```python
from build123d import *


with BuildPart() as part:
    # Sketch1 → Revolve1 (revolve)
    with BuildSketch(Plane.XY, mode=Mode.PRIVATE) as revolve1_sk:
        with BuildLine():
            Line((0, 0), (55.850610629, 0))
            ThreePointArc((55.850610629, 0), (64.83086675, 3.719743879), (68.550610629, 12.7))
            Line((68.550610629, 12.7), (68.550610629, 135.537090781))
            ThreePointArc((68.550610629, 135.537090781), (67.07437947, 141.479902659), (62.988876295, 146.041145392))
            Line((62.988876295, 146.041145392), (36.426242146, 164.092378593))
            ThreePointArc((36.426242146, 164.092378593), (33.255344861, 167.632513451), (32.109591896, 172.244930881))
            Line((32.109591896, 172.244930881), (32.109591896, 182.693006016))
            Line((32.109591896, 182.693006016), (37.812538782, 182.693006016))
            Line((37.812538782, 182.693006016), (37.812538782, 191.889991998))
            Line((37.812538782, 191.889991998), (0, 191.889991998))
            Line((0, 191.889991998), (0, 0))
        make_face()
    revolve(revolve1_sk.sketch.rotate(Axis((0, 191.889991998, 0), (0, -1, 0)), 90), axis=Axis((0, 191.889991998, 0), (0, -1, 0)))


solid = part.part
```
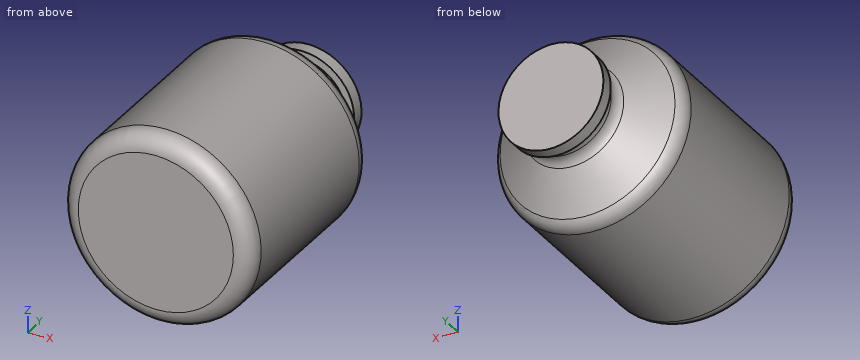
Build history of the part. All positions in model axes, mm. Coordinates: 2 decimals unless noted, no trailing zeros. Order: outer loops, then holes, each group sorted by start corner. A loop starts at its lowest first (then second) coordinate and runs counter-clockwise, first axis right, second up.
Item 1: Saw through at B-B on z = 0. List the corners of the cut face in (x, y), then the cut area to 3 significant figures.
Filled in:
outline: (-68.55, 12.7) arc R12.7 ccw to (-55.85, 0) - (55.85, 0) arc R12.7 ccw to (68.55, 12.7) - (68.55, 135.54) arc R12.7 ccw to (62.99, 146.04) - (36.43, 164.09) arc R9.86 cw to (32.11, 172.24) - (32.11, 182.69) - (37.81, 182.69) - (37.81, 191.89) - (-37.81, 191.89) - (-37.81, 182.69) - (-32.11, 182.69) - (-32.11, 172.24) arc R9.86 cw to (-36.43, 164.09) - (-62.99, 146.04) arc R12.7 ccw to (-68.55, 135.54) - close
area: 23,600 mm2
Item 2: Drop flat-ended pins along their axis: pin 1 Ø6 at (x, y) = (21.5, 164) entering from -Z; pin 2 Ø2 at (y, z) = (145, -9) entering from -X; pin 3 Ø12 at (x, z) = (-50.5, 19.5) entering from -Y; pin 4 Ø4 at (x, y) = (41, 30) entering from +Z. Give the stop position or say it passes through.
Filled in:
pin 1: stops at z = -35.19
pin 2: stops at x = -64.71
pin 3: stops at y = 0
pin 4: stops at z = 56.38
Item 3: Saw through at A-A on x = 0. List the corners of the cut face in (y, z).
Filled in:
outline: (0, -55.85) arc R12.7 ccw to (12.7, -68.55) - (135.54, -68.55) arc R12.7 ccw to (146.04, -62.99) - (164.09, -36.43) arc R9.86 cw to (172.24, -32.11) - (182.69, -32.11) - (182.69, -37.81) - (191.89, -37.81) - (191.89, 37.81) - (182.69, 37.81) - (182.69, 32.11) - (172.24, 32.11) arc R9.86 cw to (164.09, 36.43) - (146.04, 62.99) arc R12.7 ccw to (135.54, 68.55) - (12.7, 68.55) arc R12.7 ccw to (0, 55.85) - close
Item 4: Drill centre lines: L1, parallel to Y at x = 19, z = -31; L2, parallel to Z at x = 10.5, y = 102; L3, parallel to Z at x = 7, y = 167. Where is each one in solid material? Low to high.
Filled in:
L1: y = 0 to 164.14, 182.69 to 191.89
L2: z = -67.74 to 67.74
L3: z = -32.88 to 32.88
Item 5: Saw through at C-C on y = 57. List the corners of the cut face in (x, z).
Filled in:
outline: circle Ø137.1 at (0, 0)
